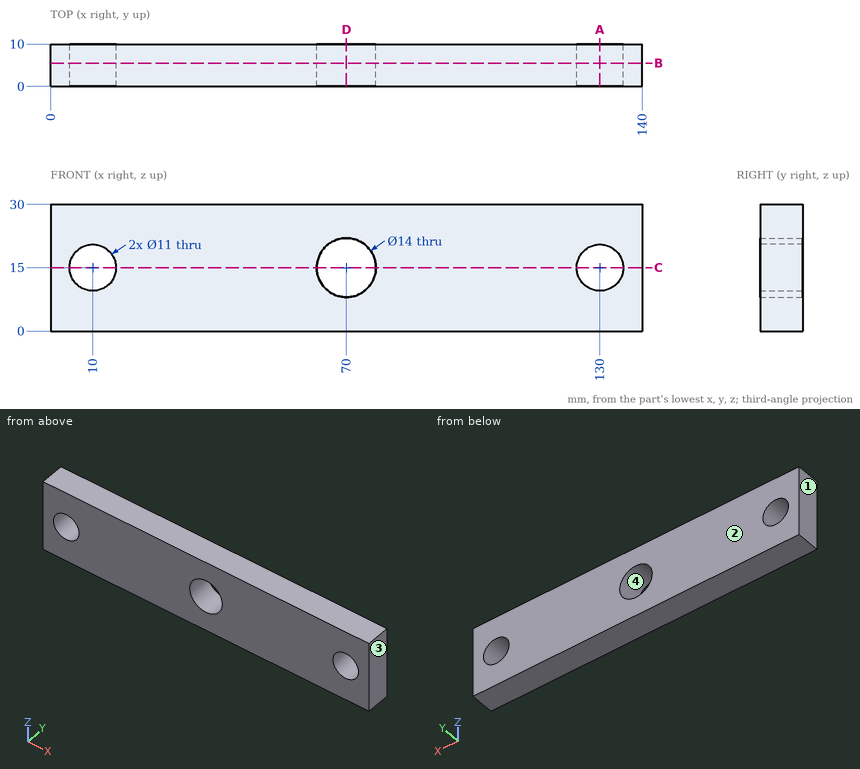
Answer from the drawing. Dimensions are ordinates in mm from the lowest x, y and z of the part. Give positions to 0.01 mm unless a question says otherwise; leave off trailing zeros. Order: outer loops, then holes, each group sorted by start corner. A loop starts at its lowest first (then second) coordinate and runs counter-clockwise, first axis right, second up. Notation, with made-up numbers: (20, 77) -> (64, 77) arc R18 ccw to (64, 101) -> close; hole circle Ø11 at (26, 13.25). An arc over 180 degrees is marked (long way). One line per item, written item: value.
Item 1: Find section B-B, the plane y = 5.5. Give the vertices of the cut face in (x, z).
Answer sheet:
outline: (0, 0) -> (140, 0) -> (140, 30) -> (0, 30) -> close; hole circle Ø11 at (10, 15); hole circle Ø14 at (70, 15); hole circle Ø11 at (130, 15)
Item 2: Find section D-D, the plane x = 70. Give the vertices of the cut face in (y, z).
Answer sheet:
outline: (0, 0) -> (10, 0) -> (10, 8) -> (0, 8) -> close; (0, 22) -> (10, 22) -> (10, 30) -> (0, 30) -> close
Item 3: Find section C-C, the plane z = 15. Give the vertices of the cut face in (x, y), plus the area to 3 significant figures.
Answer sheet:
outline: (0, 0) -> (4.5, 0) -> (4.5, 10) -> (0, 10) -> close; (15.5, 0) -> (63, 0) -> (63, 10) -> (15.5, 10) -> close; (77, 0) -> (124.5, 0) -> (124.5, 10) -> (77, 10) -> close; (135.5, 0) -> (140, 0) -> (140, 10) -> (135.5, 10) -> close
area: 1,040 mm²
Item 4: Find section A-A, the plane x = 130. Give the vertices of the cut face in (y, z).
Answer sheet:
outline: (0, 0) -> (10, 0) -> (10, 9.5) -> (0, 9.5) -> close; (0, 20.5) -> (10, 20.5) -> (10, 30) -> (0, 30) -> close
Item 5: Determine the mould class of the marked faces 1, 2, 3 and 4 for opening direction X: released by +X, released by -X, zero draft, split by the parting line, or undercut.
Answer sheet:
face 1: released by -X
face 2: zero draft
face 3: released by +X
face 4: undercut
Item 6: Straight lines are drawn through the part: probe 1 along X at (y, z) = (7.25, 15); probe 2 along X at (y, z) = (7, 13); probe 3 along Z at (x, y) = (70, 3.75). For each, find the intervals that lie inside material, in ascending order.
Answer sheet:
probe 1: 0 to 4.5, 15.5 to 63, 77 to 124.5, 135.5 to 140
probe 2: 0 to 4.88, 15.12 to 63.29, 76.71 to 124.88, 135.12 to 140
probe 3: 0 to 8, 22 to 30
